from build123d import *

# Parameters (mm, degrees)
SKETCH1_W           = 39
SKETCH1_H           = 13
BOSS_EXTRUDE1_DEPTH = 2
SKETCH3_W           = 2
SKETCH3_H           = 13
SKETCH3_W_2         = 4.8
BOSS_EXTRUDE2_DEPTH = 1
SKETCH4_W           = 14.8
SKETCH4_H           = 13
SKETCH4_W_2         = 12
BOSS_EXTRUDE3_DEPTH = 2
SKETCH5_W           = 23
SKETCH5_H           = 11.8
CUT_EXTRUDE1_DEPTH  = 31.356218473
SKETCH6_R           = 1
BOSS_EXTRUDE4_DEPTH = 3
SKETCH7_W           = 32.2
SKETCH7_H           = 0.6
BOSS_EXTRUDE5_DEPTH = 10
SKETCH8_W           = 2
SKETCH8_H           = 13
BOSS_EXTRUDE6_DEPTH = 7


with BuildPart() as part:
    # Sketch1 → Boss-Extrude1 (new body)
    with BuildSketch(Plane(origin=(0, 0, 0), x_dir=(1, 0, 0), z_dir=(0, 1, 0))):
        Rectangle(SKETCH1_W, SKETCH1_H)
    extrude(amount=BOSS_EXTRUDE1_DEPTH)

    # Sketch3 → Boss-Extrude2 (add)
    with BuildSketch(Plane(origin=(0, 2, 0), x_dir=(1, 0, 0), z_dir=(0, 1, 0))):
        with Locations((18.5, 0)):
            Rectangle(SKETCH3_W, SKETCH3_H)
        with Locations((-17.1, 0)):
            Rectangle(SKETCH3_W_2, SKETCH3_H)
    extrude(amount=BOSS_EXTRUDE2_DEPTH)

    # Sketch4 → Boss-Extrude3 (add)
    with BuildSketch(Plane(origin=(0, 3, 0), x_dir=(1, 0, 0), z_dir=(0, 1, 0))):
        with Locations((-22.1, 0)):
            Rectangle(SKETCH4_W, SKETCH4_H)
        with Locations((23.5, 0)):
            Rectangle(SKETCH4_W_2, SKETCH4_H)
    extrude(amount=BOSS_EXTRUDE3_DEPTH)

    # Sketch5 → Cut-Extrude1 (cut, through all)
    with BuildSketch(Plane(origin=(0, 2, 0), x_dir=(1, 0, 0), z_dir=(0, 1, 0))):
        with Locations((1.4, 0)):
            Rectangle(SKETCH5_W, SKETCH5_H)
    extrude(amount=-CUT_EXTRUDE1_DEPTH, mode=Mode.SUBTRACT)

    # Sketch6 → Boss-Extrude4 (add)
    with BuildSketch(Plane(origin=(0, 2, 0), x_dir=(1, 0, 0), z_dir=(0, 1, 0))):
        with Locations(Location((-12.4, 0, 0), (0, 0, 270))):
            Circle(SKETCH6_R)
        with Locations(Location((15.2, 0, 0), (0, 0, 270))):
            Circle(SKETCH6_R)
    extrude(amount=BOSS_EXTRUDE4_DEPTH)

    # Sketch7 → Boss-Extrude5 (add)
    with BuildSketch(Plane(origin=(0, 2, 0), x_dir=(1, 0, 0), z_dir=(0, 1, 0))):
        with Locations((1.4, -6.2)):
            Rectangle(SKETCH7_W, SKETCH7_H)
        with Locations((1.4, 6.2)):
            Rectangle(SKETCH7_W, SKETCH7_H)
    extrude(amount=BOSS_EXTRUDE5_DEPTH)

    # Sketch8 → Boss-Extrude6 (add)
    with BuildSketch(Plane(origin=(0, 5, 0), x_dir=(1, 0, 0), z_dir=(0, 1, 0))):
        with Locations((-15.7, 0)):
            Rectangle(SKETCH8_W, SKETCH8_H)
        with Locations((18.5, 0)):
            Rectangle(SKETCH8_W, SKETCH8_H)
    extrude(amount=BOSS_EXTRUDE6_DEPTH)


solid = part.part
Input: part model. Units: mm. Frame: model coordinates. A direction names the side the tool comes from. Give positions to 0.01 mm unless a question says otherwise; leave off trailing zeros. Order: outer loops, then holes, each group sorted by start corner. A loop starts at its lowest first (then second) coordinate and runs counter-clockwise, first axis right, second up. Notation, with made-up numbers: (45.5, 84.25) -> (75.5, 84.25) arc R13 cw to (75.5, 103.25) -> close; hole circle Ø4 at (49, 43). An arc over 180 degrees is marked (long way). Use one line per item in the form item = value.
1) Section C-C, the plane y = 7.5. Return loops of the section in (x, z), and give its area (3 significant figures).
Response values:
outline = (-16.7, -6.5) -> (19.5, -6.5) -> (19.5, 6.5) -> (-16.7, 6.5) -> close; hole (-14.7, -5.9) -> (17.5, -5.9) -> (17.5, 5.9) -> (-14.7, 5.9) -> close
area = 90.6 mm^2
2) Line query: probe 1 along X at (y, z) = (4.25, 2); probe 2 along Z at (x, y) = (-8.5, 9); probe 3 along X at (y, z) = (2.5, 4.25). Output: solid intervals per line, ascending.
Response values:
probe_1 = -29.5 to -14.7, 17.5 to 29.5
probe_2 = -6.5 to -5.9, 5.9 to 6.5
probe_3 = -19.5 to -14.7, 17.5 to 19.5
3) Mould query, pull axis Z, two halves, no side actions, for faces 6 (the flat face through (-12.4, 2, -1.4)), 7 (the flat face through (0, 6, 6.5)), 8 (the flat face through (-19.5, 1, 0)), 9 (the cylindrical face through (-13.376, 3.479, -0.217)). Classes: pulls with the +Z half, pulls with the -Z half, needs draft (parallel to the pull), parting line crosses it, or undercut.
Response values:
face_6 = undercut
face_7 = pulls with the +Z half
face_8 = needs draft
face_9 = undercut
4) Reachability of faces 1 (the flat face through (-23, 5, 0)), 2 (the flat face through (12.9, 1, 0)), 3 (the flat face through (19.5, 8, 0)), 4 (the flat face through (15, 5, 0)), 5 (the flat face through (24, 3, 0)) from +Z, -Z, +X, -X, +Y, -Y: full face, straight path, thin tool, end or side. Return the list, or none.
Response values:
face_1 = +Z, -Z, -X, +Y
face_2 = +Y, -Y
face_3 = +Z, -Z, +X, +Y
face_4 = +Y
face_5 = +Z, -Z, +X, -Y
5) First-contact query: pin 1 Ø1.6 at (x, z) = (15, 0) entering from +Y; pin 2 Ø6 at (x, z) = (21, 0.5) entering from -Y; pin 3 Ø3 at (x, z) = (-26, -2) entering from -Y; pin 4 Ø3.5 at (y, z) = (1, 3) entering from -X. Flat tips, straight axial feed; report the tip coordinate or a pass-through.
Response values:
pin_1 = 5
pin_2 = 0
pin_3 = 3
pin_4 = -19.5
6) Section B-B, the plane z = 2. Return loops of the section in (x, y), and give its area (3 significant figures).
Response values:
outline = (-29.5, 3) -> (-19.5, 3) -> (-19.5, 0) -> (-10.1, 0) -> (-10.1, 2) -> (-14.7, 2) -> (-14.7, 12) -> (-16.7, 12) -> (-16.7, 5) -> (-29.5, 5) -> close; (12.9, 0) -> (19.5, 0) -> (19.5, 3) -> (29.5, 3) -> (29.5, 5) -> (19.5, 5) -> (19.5, 12) -> (17.5, 12) -> (17.5, 2) -> (12.9, 2) -> close
area = 120 mm^2
7) Section A-A, the plane y = 3.5. Return loops of the section in (x, z).
Response values:
outline = (-29.5, -6.5) -> (29.5, -6.5) -> (29.5, 6.5) -> (-29.5, 6.5) -> close; circle Ø2 at (-12.4, 0); circle Ø2 at (15.2, 0); hole (-14.7, -5.9) -> (17.5, -5.9) -> (17.5, 5.9) -> (-14.7, 5.9) -> close
8) Section D-D, the plane x = 15.2. Return loops of the section in (y, z), and give its area (3 significant figures).
Response values:
outline = (0, -6.5) -> (12, -6.5) -> (12, -5.9) -> (2, -5.9) -> (2, -1) -> (5, -1) -> (5, 1) -> (2, 1) -> (2, 5.9) -> (12, 5.9) -> (12, 6.5) -> (0, 6.5) -> close
area = 44.0 mm^2
